```python
from build123d import *

# Parameters (mm, degrees)
CHANFRO1_SIZE = 1
CHANFRO3_SIZE = 2
CHANFRO4_SIZE = 5


with BuildPart() as part:
    # Esboço1 → Revolução1 (revolve)
    with BuildSketch(Plane(origin=(0, 0, 0), x_dir=(0, 0, -1), z_dir=(1, 0, 0))):
        Polygon((0.5, 12), (0.5, 19.5), (12.5, 19.5), (12.5, 18), (15.5, 18), (15.5, 19.9), (56.6, 19.9), (60.5, 16), (70.5, 16), (72, 17.5), (80.5, 17.5), (80.5, 12), (80.5, 11), (63.5, 11), (63.5, 12), align=None)
    revolve(axis=Axis((0, 0, 0), (0, 0, -1)))

    # Chanfro1
    chanfro1_edges = [part.edges().sort_by_distance(p)[0] for p in [
        (0, -19.5, -0.5),
        (0, -19.5, -12.5),
    ]]
    chamfer(chanfro1_edges, length=CHANFRO1_SIZE)

    # Chanfro3
    chanfro3_edges = [part.edges().sort_by_distance(p)[0] for p in [
        (0, -11, -80.5),
    ]]
    chamfer(chanfro3_edges, length=CHANFRO3_SIZE)

    # Chanfro4
    chanfro4_edges = [part.edges().sort_by_distance(p)[0] for p in [
        (0, -12, -0.5),
    ]]
    chamfer(chanfro4_edges, length=CHANFRO4_SIZE)


solid = part.part
```
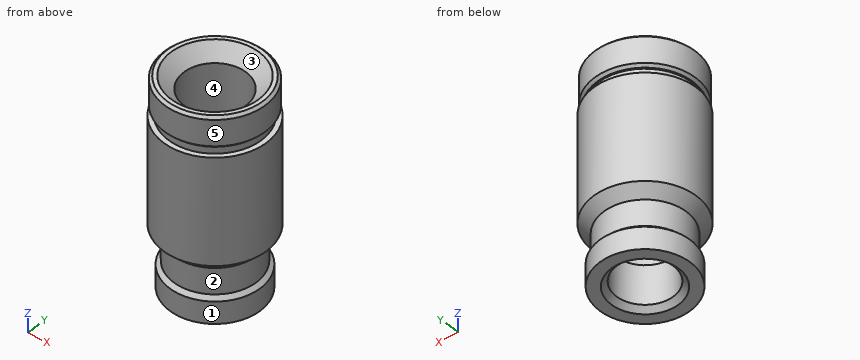
Design review of the part built by this model. Coordinates are the model's own, in mm. Face numbers are marked on the shaded views. A direction names the side the tool comes from. Coordinates: 2 decimals unless noted, no trailing zeros. Order: outer loops, then holes, each group sorted by start corner. A loop starts at its lowest first (then second) coordinate and runs counter-clockwise, first axis right, second up.
1) Take a section at B-B, the plane z = -68. Give the boundary of the cut face in (x, y).
2) For the marked faces 1, 2 and 3, list the 3-axis set-ups (+Z, -Z, +X, -X, +Y, -Y) from which the entire face can be reached by the end or side of a thin tool; tool diameter is ignored.
3) Wall thickness on line 1 along X through (y, z) = (0, -69.5); line 2 along X through (y, z) = (0, -50); line 3 along Z through (x, y) = (12, -14.5): over which ranges is each line inside the solid? List them lowest first.
4) Clearance check with flat-ended pins moving along their axes: pin 1 (3 mm diameter, centred on x = 14.5, z = -33.5, fed in from -Y); pin 2 (5 mm diameter, centred on x = 6, z = -23.5, fed in from +Y); pin 3 (11 mm diameter, centred on x = 7, y = -8, fed in from -Z); pin 4 (6 mm diameter, centred on y = 15, z = -39, fed in from -X). State where each tip first meets the part, or that it passes through.
5) Mouldability with a two-part tool opening along Y and no side actions: class the marked faces 4 and 5 as +Y half, -Y half, draft (parallel to the pull), parting line (faces both ways), or undercut.
6) Take a section at A-A, the plane z = -39. Give the boundary of the cut face in (x, y).
Returned:
1. outline: circle Ø32 at (0, 0); hole circle Ø22 at (0, 0)
2. face 1: -Z
2. face 2: none
2. face 3: +Z
3. line 1: x = -16 to -11, 11 to 16
3. line 2: x = -19.9 to -12, 12 to 19.9
3. line 3: z = -57.68 to -15.5, -12.18 to -0.82
4. pin 1: stops at y = -15.07
4. pin 2: stops at y = 19.59
4. pin 3: stops at z = -80.5
4. pin 4: stops at x = -15.87
5. face 4: undercut
5. face 5: parting line
6. outline: circle Ø39.8 at (0, 0); hole circle Ø24 at (0, 0)
